from build123d import *

# Parameters (mm, degrees)
F0_W      = 90
F0_H      = 80
F1_DEPTH  = 4
F2_R      = 1.5
F3_DEPTH  = 4.001
F5_DEPTH  = 14
F6_W      = 7
F6_H      = 15
F7_DEPTH  = 2
F8_W      = 3.75
F8_H      = 60
F9_DEPTH  = 2
F10_W     = 3.75
F10_H     = 15
F10_W_2   = 3.25
F11_DEPTH = 3
F12_W     = 3.75
F12_H     = 45
F13_DEPTH = 16.001
F14_W     = 19
F14_H     = 1.5
F15_DEPTH = 25
F16_W     = 3.75
F16_H     = 22.5
F17_DEPTH = 25
F18_W     = 32
F18_H     = 2
F19_DEPTH = 1.5
F20_R     = 1
F21_W     = 1.4166666667
F21_H     = 32
F22_DEPTH = 0.7085
F23_SIZE  = 0.7075
F24_SIZE  = 1.8
F25_W     = 3.75
F25_H     = 7.5
F25_W_2   = 60.0602255464
F25_H_2   = 3.75
F26_DEPTH = 25
F27_W     = 15.25
F27_H     = 32
F28_DEPTH = 1.5
F29_W     = 32
F29_H     = 13.5
F30_DEPTH = 0.3
F31_W     = 3.25
F31_H     = 15
F32_DEPTH = 1.3
F33_W     = 15
F33_H     = 10.7
F34_DEPTH = 0.3
F35_W     = 1.2
F35_H     = 32
F36_DEPTH = 1
F37_R     = 1.19999


# Not quite as in the source:
# - a fillet or chamfer is up to 0.001 mm smaller than in the source, because OpenCascade refuses the exact size
# - a feature names something its author has since deleted; it is built from what else it names


with BuildPart() as f1:
    # F0 (on Top) → F1 (new body)
    with BuildSketch(Plane.XY):
        Rectangle(F0_W, F0_H)
    extrude(amount=F1_DEPTH)

    # F2 (on face) → F3 (cut, through all)
    with BuildSketch(Plane.XY.offset(4)):
        with Locations((23, 0)):
            Circle(F2_R)
        with Locations((-15, 0)):
            Circle(F2_R)
    extrude(amount=-F3_DEPTH, mode=Mode.SUBTRACT)

    # F4 (on face) → F5 (join)
    with BuildSketch(Plane(origin=(0, 0, 0), x_dir=(1, 0, 0), z_dir=(0, 0, -1))):
        Polygon((-41.25, -36.25), (-41.25, 36.25), (-30, 36.25), (-30, 40), (-45, 40), (-45, -40), (-41.25, -40), align=None)
        Polygon((45, 40), (30, 40), (30, 36.25), (41.25, 36.25), (41.25, -36.25), (41.25, -40), (45, -40), align=None)
    extrude(amount=F5_DEPTH)

    # F6 (on face) → F7 (join)
    with BuildSketch(Plane(origin=(0, 0, -14), x_dir=(1, 0, 0), z_dir=(0, 0, -1))):
        with Locations((41.5, 32.5)):
            Rectangle(F6_W, F6_H)
    extrude(amount=F7_DEPTH)

    # F8 (on face) → F9 (cut)
    with BuildSketch(Plane(origin=(0, 0, -14), x_dir=(1, 0, 0), z_dir=(0, 0, -1))):
        with Locations((43.125, -10)):
            Rectangle(F8_W, F8_H)
    extrude(amount=-F9_DEPTH, mode=Mode.SUBTRACT)

    # F10 (on face) → F11 (join)
    with BuildSketch(Plane(origin=(0, 0, -12), x_dir=(1, 0, 0), z_dir=(0, 0, -1))):
        with Locations((43.125, -32.5)):
            Rectangle(F10_W, F10_H)
        with Locations((39.625, -32.5)):
            Rectangle(F10_W_2, F10_H)
    extrude(amount=F11_DEPTH)

    # F12 (on face) → F13 (cut, through all)
    with BuildSketch(Plane(origin=(0, 0, -12), x_dir=(1, 0, 0), z_dir=(0, 0, -1))):
        with Locations((43.125, -2.5)):
            Rectangle(F12_W, F12_H)
    extrude(amount=-F13_DEPTH, mode=Mode.SUBTRACT)

    # F14 (on face) → F15 (cut)
    with BuildSketch(Plane(origin=(0, 0, -14), x_dir=(1, 0, 0), z_dir=(0, 0, -1))):
        with Locations((-35.5, 16.75)):
            Rectangle(F14_W, F14_H)
        with Locations((-35.5, -16.75)):
            Rectangle(F14_W, F14_H)
    extrude(amount=-F15_DEPTH, mode=Mode.SUBTRACT)

    # F16 (on face) → F17 (cut)
    with BuildSketch(Plane(origin=(0, 0, -14), x_dir=(1, 0, 0), z_dir=(0, 0, -1))):
        with Locations((-43.125, -28.75)):
            Rectangle(F16_W, F16_H)
    extrude(amount=-F17_DEPTH, mode=Mode.SUBTRACT)

    # F18 (on face) → F19 (join)
    with BuildSketch(Plane.YZ.offset(-41.25)):
        with Locations((0, -13)):
            Rectangle(F18_W, F18_H)
    extrude(amount=F19_DEPTH)

    # F20
    f20_edges = [f1.edges().sort_by_distance(p)[0] for p in [
        (-39.75, 0, -14),
    ]]
    fillet(f20_edges, radius=F20_R)

    # F21 (on face) → F22 (join)
    with BuildSketch(Plane(origin=(0, 0, -14), x_dir=(1, 0, 0), z_dir=(0, 0, -1))):
        with Locations((-41.4583333333, 0)):
            Rectangle(F21_W, F21_H)
        with Locations((-44.2916666667, 0)):
            Rectangle(F21_W, F21_H)
    extrude(amount=F22_DEPTH)

    # F23 (size 0.7085 in the source; OpenCascade refuses exactly that, so slightly less here)
    f23_edges = [f1.edges().sort_by_distance(p)[0] for p in [
        (-40.75, 0, -14.7085),
        (-42.166667, 0, -14.7085),
        (-43.583333, 0, -14.7085),
        (-45, 0, -14.7085),
    ]]
    chamfer(f23_edges, length=F23_SIZE)

    # F24
    f24_edges = [f1.edges().sort_by_distance(p)[0] for p in [
        (-16.5, 0, 0),
        (21.5, 0, 0),
    ]]
    chamfer(f24_edges, length=F24_SIZE)

    # F25 (on face) → F26 (cut)
    with BuildSketch(Plane(origin=(0, 0, -14), x_dir=(1, 0, 0), z_dir=(0, 0, -1))):
        with Locations((-43.125, 21.25)):
            Rectangle(F25_W, F25_H)
        with Locations((0.0301127732, 38.125)):
            Rectangle(F25_W_2, F25_H_2)
    extrude(amount=-F26_DEPTH, mode=Mode.SUBTRACT)

    # F27 (on face) → F28 (cut)
    with BuildSketch(Plane(origin=(0, 0, 0), x_dir=(1, 0, 0), z_dir=(0, 0, -1))):
        with Locations((-33.625, 0)):
            Rectangle(F27_W, F27_H)
    extrude(amount=-F28_DEPTH, mode=Mode.SUBTRACT)

    # F29 (on face) → F30 (join)
    with BuildSketch(Plane.YZ.offset(-41.25)):
        with Locations((0, -5.25)):
            Rectangle(F29_W, F29_H)
    extrude(amount=F30_DEPTH)

    # F31 (on face) → F32 (join)
    with BuildSketch(Plane.XY.offset(-12)):
        with Locations((39.625, 32.5)):
            Rectangle(F31_W, F31_H)
    extrude(amount=F32_DEPTH)

    # F33 (on face) → F34 (join)
    with BuildSketch(Plane(origin=(41.25, 0, 0), x_dir=(0, -1, 0), z_dir=(-1, 0, 0))):
        with Locations((-32.5, -5.35)):
            Rectangle(F33_W, F33_H)
    extrude(amount=F34_DEPTH)

    # F35 (on face) → F36 (join)
    with BuildSketch(Plane.XY.offset(-12)):
        with Locations((-40.35, 0)):
            Rectangle(F35_W, F35_H)
    extrude(amount=F36_DEPTH)

    # F37 (radius 1.2 in the source; OpenCascade refuses exactly that, so slightly less here)
    f37_edges = [f1.edges().sort_by_distance(p)[0] for p in [
        (-39.75, 0, -11),
    ]]
    fillet(f37_edges, radius=F37_R)


solid = f1.part
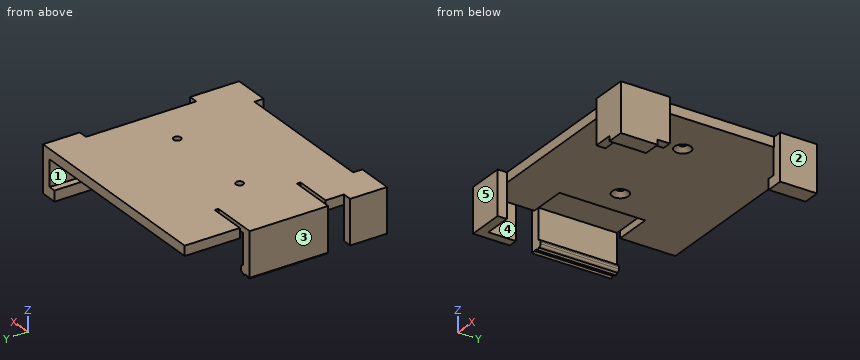
Geometry check sheet. Reference: the model listing, model coordinates, mm. Face numbers are marked on the shaded views. A direction names the side the tool comes from. Give positions to 0.01 mm unless a question says otherwise; leave off trailing zeros. Order: outer loops, then holes, each group sorted by start corner. A loop starts at its lowest first (then second) coordinate and runs counter-clockwise, first axis right, second up.
1. Sectioned sample at A-A (x = 23). Record the boundary of the cut face in (y, z), then the cut area to 3 significant figures.
Completed:
outline: (-36.25, 0) - (-3.3, 0) - (-1.5, 1.8) - (-1.5, 4) - (-36.25, 4) - close; (1.5, 1.8) - (3.3, 0) - (40, 0) - (40, 4) - (1.5, 4) - close
area: 290 mm2
2. Access from +Z, -Z, +X, -X, +Y, -Y to the whole of each face (thin tool, end or side, straight path). Record for the marked faces 1 and 2.
Completed:
face 1: -X, +Y
face 2: +Z, -Z, +X, +Y, -Y
3. Depth check by flat-ended pin: pin 1 (0.6 mm diameter, centred on y = -32, z = -14.5, fed in from -X); pin 2 (4 mm diameter, centred on x = -10, z = 1, fed in from -Y); pin 3 (1.9 mm diameter, centred on x = 43, y = -23, fed in from -Z). Enter the tip coordinate at first touch or a pass-through.
Completed:
pin 1: stops at x = 38
pin 2: stops at y = -36.25
pin 3: stops at z = -14
4. Scan lines: line 1 (Y direction, x = -15, z = 3.35); line 2 (Y direction, x = 35, z = -3); line 3 (X direction, y = -6, z = 0.75). Record each from-to range of solid material in increasing order.
Completed:
line 1: y = -36.25 to -1.5, 1.5 to 40
line 2: y = -40 to -36.25
line 3: x = -45 to -40.95, -26 to 41.25
5. Sectioned sample at C-C (x = -35.5). Record the boundary of the cut face in (y, z), then the cut area to 4 significant figures.
Completed:
outline: (-40, -14) - (-36.25, -14) - (-36.25, 0) - (-17.5, 0) - (-17.5, 4) - (-40, 4) - close; (-16, 1.5) - (16, 1.5) - (16, 4) - (-16, 4) - close; (17.5, 0) - (40, 0) - (40, 4) - (17.5, 4) - close
area: 312.5 mm2
6. Draft check along Y on the marked faces 3, 4 and 5. Enter one of: pulls with the +Y half, pulls with the -Y half, needs draft (parallel to the pull), parting line crosses it, or undercut.
Completed:
face 3: needs draft
face 4: undercut
face 5: pulls with the -Y half
7. Sectioned sample at B-B (y = 0). State how many separate pieces and enclosed holes the cut face has, then the cut area to 3 significant figures.
Completed:
separate pieces: 3
enclosed holes: 0
area: 353 mm2
